Build history of the part. All positions in model axes, mm. Face numbers are marked on the shaded views. A direction names the side the tool comes from. Coordinates: 2 decimals unless noted, no trailing zeros. Order: outer loops, then holes, each group sorted by start corner. A loop starts at its lowest first (then second) coordinate and runs counter-clockwise, first axis right, second up. Notation, with made-up numbers: (86.5, 34.25) - (109.5, 34.25) arc R12 cw to (109.5, 57.25) - close; hole circle Ø5 at (-0.75, 29). An arc over 180 degrees is marked (long way). One line per item, written item: value.
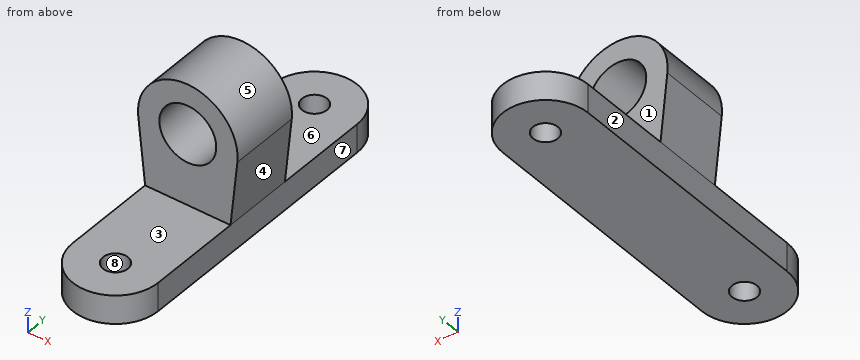
from build123d import *

# Parameters (mm, degrees)
ESBO_O1_R                = 1.75
RESSALTO_EXTRUS_O1_DEPTH = 4
ESBO_O2_W                = 32.967162932
ESBO_O2_H                = 10
RESSALTO_EXTRUS_O2_DEPTH = 25
ESBO_O3_R                = 4
CORTE_EXTRUS_O3_DEPTH    = 42.895088709


with BuildPart() as part:
    # Esboço1 → Ressalto-extrusão1 (new body)
    with BuildSketch(Plane.XY):
        with BuildLine():
            Line((-6, 0), (-6, 36.6))
            ThreePointArc((-6, 36.6), (0, 42.6), (6, 36.6))
            Line((6, 36.6), (6, 0))
            ThreePointArc((6, 0), (0, -6), (-6, 0))
        make_face()
        Circle(ESBO_O1_R, mode=Mode.SUBTRACT)
        with Locations((0, 36.6)):
            Circle(ESBO_O1_R, mode=Mode.SUBTRACT)
    extrude(amount=RESSALTO_EXTRUS_O1_DEPTH)

    # Esboço2 → Ressalto-extrusão2 (add)
    with BuildSketch(Plane(origin=(0, 0, 0), x_dir=(-1, 0, 0), z_dir=(0, 0, -1))):
        with Locations((0, 18.3)):
            Rectangle(ESBO_O2_W, ESBO_O2_H)
    extrude(amount=-RESSALTO_EXTRUS_O2_DEPTH)

    # Esboço3 → Corte-extrusão3 (cut, through all)
    with BuildSketch(Plane(origin=(0, 23.3, 0), x_dir=(1, 0, 0), z_dir=(0, 1, 0))):
        with BuildLine():
            Line((-6.962621571, -13.277572943), (-6, -4))
            Line((-6, -4), (-6, 0))
            Line((-6, 0), (-16.483581466, 0))
            Line((-16.483581466, 0), (-16.483581466, -25))
            Line((-16.483581466, -25), (16.483581466, -25))
            Line((16.483581466, -25), (16.483581466, 0))
            Line((16.483581466, 0), (6, 0))
            Line((6, 0), (6, -4))
            Line((6, -4), (6.962621571, -13.277572943))
            ThreePointArc((6.962621571, -13.277572943), (0, -21), (-6.962621571, -13.277572943))
        make_face()
        with Locations(Location((0, -14, 0), (0, 0, 270))):
            Circle(ESBO_O3_R)
    extrude(amount=-CORTE_EXTRUS_O3_DEPTH, mode=Mode.SUBTRACT)


solid = part.part
1. Probe line 1 along Y through (x, z) = (0, 3.25); line 2 along X through (y, z) = (19.5, 14); line 3 along Y through (x, z) = (3.25, 10.25). List the from-to ranges inside material, lowest first.
Values found:
line 1: y = -6 to -1.75, 1.75 to 34.85, 38.35 to 42.6
line 2: x = -7 to -4, 4 to 7
line 3: y = 13.3 to 23.3
2. Band-saw the part on C-C, the plane x = -2.25. Give the cut face in (y, z).
Values found:
outline: (-5.56, 0) - (42.16, 0) - (42.16, 4) - (23.3, 4) - (23.3, 10.69) - (13.3, 10.69) - (13.3, 4) - (-5.56, 4) - close; (13.3, 17.31) - (23.3, 17.31) - (23.3, 20.63) - (13.3, 20.63) - close
3. Band-saw the part on D-D, the plane y = 2.5. Give the cut face in (x, z), and give its area (3 significant figures).
Values found:
outline: (-6, 0) - (6, 0) - (6, 4) - (-6, 4) - close
area: 48.0 mm2
4. Two-plate mould, pull along X, no slides. Class the marked faces 5, 6, 7 and 8: pulls with the +X half, pulls with the -X half, needs draft (parallel to the pull), parting line crosses it, or undercut.
Values found:
face 5: parting line crosses it
face 6: needs draft
face 7: pulls with the +X half
face 8: undercut
5. Flat gauge pins, fed straight in: P1, Ø2, axis at y = 15.5, z = 1.5, coming from the +X side; P2, Ø1, axis at x = 3, y = 32.5, coming from the +Z side; P3, Ø7, axis at x = 0, z = 16, coming from the +Y side. Where does each tip first touch, or does it go through?
Values found:
P1: stops at x = 6
P2: stops at z = 4
P3: stops at y = 23.3
6. 3-axis set-ups, long thin cutter, end or side, ignore diameter. For the marked faces 1, 2, 3 and 4: which of +Z, -Z, +X, -X, +Y, -Y reach the whole face in a straight line?
Values found:
face 1: +Z, +X, -X, +Y
face 2: -Z, -X, +Y, -Y
face 3: +Z, +X, -X, -Y
face 4: -Z, +X, +Y, -Y
7. Band-saw the part on B-B, the plane x = 0. Give the cut face in (y, z).
Values found:
outline: (-6, 0) - (-1.75, 0) - (-1.75, 4) - (-6, 4) - close; (1.75, 0) - (34.85, 0) - (34.85, 4) - (23.3, 4) - (23.3, 10) - (13.3, 10) - (13.3, 4) - (1.75, 4) - close; (13.3, 18) - (23.3, 18) - (23.3, 21) - (13.3, 21) - close; (38.35, 0) - (42.6, 0) - (42.6, 4) - (38.35, 4) - close
8. Band-saw the part on A-A, the plane z = 14. Give the cut face in (x, y), and give its area (3 significant figures).
Values found:
outline: (-7, 13.3) - (-4, 13.3) - (-4, 23.3) - (-7, 23.3) - close; (4, 13.3) - (7, 13.3) - (7, 23.3) - (4, 23.3) - close
area: 60.0 mm2
